```python
from build123d import *

# Parameters (mm, degrees)
SKETCH1_W           = 65
SKETCH1_H           = 65
BOSS_EXTRUDE1_DEPTH = 6
FILLET1_R           = 5
SKETCH2_W           = 41
SKETCH2_H           = 4
BOSS_EXTRUDE2_DEPTH = 8
FILLET2_R           = 2


with BuildPart() as part:
    # Sketch1 → Boss-Extrude1 (new body)
    with BuildSketch(Plane.XY):
        Rectangle(SKETCH1_W, SKETCH1_H)
    extrude(amount=BOSS_EXTRUDE1_DEPTH)

    # Fillet1
    fillet1_edges = [part.edges().sort_by_distance(p)[0] for p in [
        (32.5, -32.5, 3),
        (-32.5, -32.5, 3),
        (-32.5, 32.5, 3),
        (32.5, 32.5, 3),
    ]]
    fillet(fillet1_edges, radius=FILLET1_R)

    # Sketch2 → Boss-Extrude2 (add)
    with BuildSketch(Plane.XY.offset(6)):
        with Locations((0, -30.5)):
            Rectangle(SKETCH2_W, SKETCH2_H)
    extrude(amount=BOSS_EXTRUDE2_DEPTH)

    # Fillet2
    fillet2_edges = [part.edges().sort_by_distance(p)[0] for p in [
        (-20.5, -30.5, 6),
        (20.5, -30.5, 6),
        (-20.5, -30.5, 14),
        (20.5, -30.5, 14),
    ]]
    fillet(fillet2_edges, radius=FILLET2_R)


solid = part.part
```
The listing builds one solid part. Answer for the finished solid, in the listing's coordinates (mm). A direction names the side the tool comes from. Round coordinates to 2 decimals unless told otherwise and drop trailing zeros. Write each loop counter-clockwise with the first axis right and the second up, starting at its lowest first coordinate (ties: lowest second). Pieces come first, ordered by that corner, then holes. Notation, with made-up numbers: (65, 32.25) -> (89, 32.25) arc R34 ccw to (89, 63.25) -> close; hole circle Ø10 at (77, -10). An arc over 180 degrees is marked (long way). Use CSV: the item, a comma, the result in double quotes. Start each with the question number.
(1) Which of the six approach directions +Z, -Z, +X, -X, +Y, -Y give full straight-line access (tool end or side, diameter ignored) to faces 1 (the face through (-20.5, -31, 10)), 2 (the face through (20.5, -31, 10)), 3 (the face through (0, -28.5, 10))?
(2) Section A-A on y = -26.5 is taken. Give the vertices of the cut face in (x, z).
(3) Section C-C on z = 9.75 is taken. Give the vertices of the cut face in (x, y).
(4) Consider L1, parallel to Y at x = 21, z = 6.25; L2, parallel to Z at x = -13, y = -25.5; L3, parallel to X at y = -28, z = 5. Determine where each line is inside the solid, lowest interval first. Write a range as from..to.
(5) Section B-B on x = -13 is taken. Give the vertices of the cut face in (y, z).
(6) Each of these flat-tipped pins is pushed along its axis until it touches: pin 1 (3 mm diameter, centred on y = -29.5, z = 9.5, fed in from -X); pin 2 (3 mm diameter, centred on y = -30.5, z = 11, fed in from +X). Where does it stop, or does it pass through?
A:
1,face 1,"+Z, -X, +Y, -Y"
1,face 2,"+Z, +X, +Y, -Y"
1,face 3,"+Z, +X, -X, +Y"
2,outline,"(-32.5, 0) -> (32.5, 0) -> (32.5, 6) -> (-32.5, 6) -> close"
3,outline,"(-20.5, -32.5) -> (20.5, -32.5) -> (20.5, -28.5) -> (-20.5, -28.5) -> close"
4,L1,"y = -32.5..-28.5"
4,L2,"z = 0..6"
4,L3,"x = -32.47..32.47"
5,outline,"(-32.5, 0) -> (32.5, 0) -> (32.5, 6) -> (-28.5, 6) -> (-28.5, 14) -> (-32.5, 14) -> close"
6,pin 1,"stops at x = -20.5"
6,pin 2,"stops at x = 20.5"
